```python
from build123d import *

# Parameters (mm, degrees)
SKETCH1_W            = 102
SKETCH1_H            = 33.5
BOSS_EXTRUDE1_DEPTH  = 1.7
SKETCH2_W            = 23
SKETCH2_H            = 28.1
CUT_EXTRUDE1_DEPTH   = 1.7
SKETCH4_W            = 5
SKETCH4_H            = 2.7
BOSS_EXTRUDE2_DEPTH  = 3
SKETCH5_R            = 1
CUT_EXTRUDE2_DEPTH   = 2.7
FILLET1_R            = 2
FILLET1_OF_MIRROR2_R = 2
SKETCH10_W           = 6
SKETCH10_H           = 10
CUT_EXTRUDE3_DEPTH   = 1.7


with BuildPart() as part:
    # Sketch1 → Boss-Extrude1 (new body)
    with BuildSketch(Plane(origin=(0, 0, 0), x_dir=(1, 0, 0), z_dir=(0, 1, 0))):
        Rectangle(SKETCH1_W, SKETCH1_H)
    extrude(amount=BOSS_EXTRUDE1_DEPTH)

    # Sketch2 → Cut-Extrude1 (cut)
    with BuildSketch(Plane(origin=(0, 1.7, 0), x_dir=(1, 0, 0), z_dir=(0, 1, 0))):
        with Locations((-39.5, 0)):
            Rectangle(SKETCH2_W, SKETCH2_H)
    extrude(amount=-CUT_EXTRUDE1_DEPTH, mode=Mode.SUBTRACT)

    # Sketch4 → Boss-Extrude2 (add)
    with BuildSketch(Plane(origin=(0, 1.7, 0), x_dir=(1, 0, 0), z_dir=(0, 1, 0))):
        with Locations((-48.5, -15.4)):
            Rectangle(SKETCH4_W, SKETCH4_H)
    boss_extrude2 = extrude(amount=BOSS_EXTRUDE2_DEPTH)

    # Sketch5 → Cut-Extrude2 (cut)
    with BuildSketch(Plane.XY.offset(16.75)):
        with Locations((-49, 2)):
            Circle(SKETCH5_R)
    cut_extrude2 = extrude(amount=-CUT_EXTRUDE2_DEPTH, mode=Mode.SUBTRACT)

    # Fillet1
    fillet1_edges = [part.edges().sort_by_distance(p)[0] for p in [
        (-51, 0, 15.4),
        (-51, 4.7, 15.4),
        (-46, 4.7, 15.4),
    ]]
    fillet(fillet1_edges, radius=FILLET1_R)

    # Mirror2: Boss-Extrude2, Cut-Extrude2 across plane
    add(boss_extrude2.mirror(Plane.XY))
    add(cut_extrude2.mirror(Plane.XY), mode=Mode.SUBTRACT)

    # Fillet1 of Mirror2
    fillet1_of_mirror2_edges = [part.edges().sort_by_distance(p)[0] for p in [
        (-51, 0, -15.4),
        (-51, 4.7, -15.4),
        (-46, 4.7, -15.4),
    ]]
    fillet(fillet1_of_mirror2_edges, radius=FILLET1_OF_MIRROR2_R)

    # Sketch10 → Cut-Extrude3 (cut)
    with BuildSketch(Plane(origin=(0, 1.7, 0), x_dir=(1, 0, 0), z_dir=(0, 1, 0))):
        with Locations((44, -1.25)):
            Rectangle(SKETCH10_W, SKETCH10_H)
    extrude(amount=-CUT_EXTRUDE3_DEPTH, mode=Mode.SUBTRACT)


solid = part.part
```
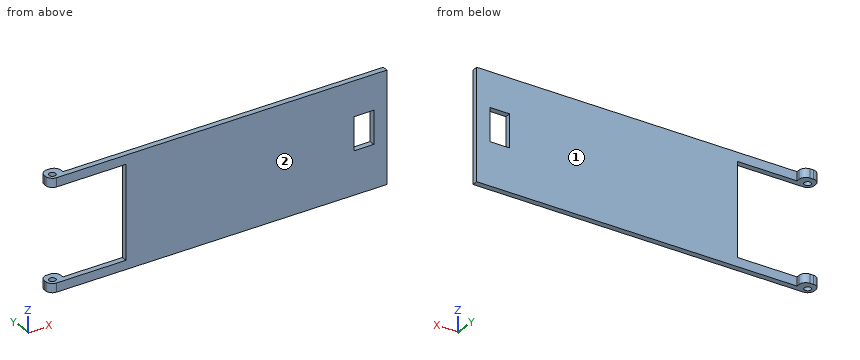
The model under review builds one solid part; all positions refer to its coordinate system, in mm. Face numbers are marked on the shaded views. A direction names the side the tool comes from. Coordinates: 2 decimals unless noted, no trailing zeros. Write each loop counter-clockwise with the first axis right and the second up, starting at its lowest first coordinate (ties: lowest second). Pieces come first, ordered by that corner, then holes.
1) To check wall thickness, follow probe 1 along X at (y, z) = (1.05, 5.5); probe 2 along Z at (x, y) = (-30, 0.5); probe 3 along Y at (x, z) = (-49, -14.65). State the ranges of each line that lie inside material, in increasing order.
2) We need section C-C on z = 15. State the section outline as (x, y) points, then the cut area to 3 significant figures.
3) We need section A-A on z = 3. State the section outline as (x, y) points, then the cut area to 3 significant figures.
4) Clearance check with flat-ended pins moving along their axes: pin 1 Ø5 at (x, z) = (19.5, 0) entering from +Y; pin 2 Ø0.8 at (y, z) = (0.5, 4) entering from -X. State where each tip first meets the part, or that it passes through.
5) We need section B-B on x = -38. State the section outline as (y, z) points.
6) We need section D-D on z = -6. State the section outline as (x, y) points, then the cut area to 3 significant figures.
7) Machinability: for the marked faces 1 and 2, which of the approach directions +Z, -Z, +X, -X, +Y, -Y give a long, thin tool a straight path to every point of the face, cutting with its end or side? Answer none if there is none.
Answer list:
1. probe 1: x = -28 to 41, 47 to 51
1. probe 2: z = -16.75 to -14.05, 14.05 to 16.75
1. probe 3: y = 0 to 1, 3 to 4.7
2. outline: (-51, 2) arc R2 ccw to (-49, 0) - (51, 0) - (51, 1.7) - (-46, 1.7) - (-46, 2.7) arc R2 ccw to (-48, 4.7) - (-49, 4.7) arc R2 ccw to (-51, 2.7) - close; hole circle Ø2 at (-49, 2)
2. area: 183 mm2
3. outline: (-28, 0) - (41, 0) - (41, 1.7) - (-28, 1.7) - close; (47, 0) - (51, 0) - (51, 1.7) - (47, 1.7) - close
3. area: 124 mm2
4. pin 1: stops at y = 1.7
4. pin 2: stops at x = -28
5. outline: (0, -16.75) - (1.7, -16.75) - (1.7, -14.05) - (0, -14.05) - close; (0, 14.05) - (1.7, 14.05) - (1.7, 16.75) - (0, 16.75) - close
6. outline: (-28, 0) - (51, 0) - (51, 1.7) - (-28, 1.7) - close
6. area: 134 mm2
7. face 1: +Z, -Z, +X, +Y
7. face 2: +Z, -Z, +X, -X, -Y
